```python
from build123d import *

# Parameters (mm, degrees)
CYLINDER100_R               = 6
CYLINDER100_DEPTH           = 9
CYLINDER020_R               = 0.8
CYLINDER020_DEPTH           = 20
ARRAY001006_X_COUNT         = 2
ARRAY001006_X_PITCH         = 22
ARRAY001006_Y_COUNT         = 2
ARRAY001006_Y_PITCH         = 22
ARRAY001006_PLACEMENT_ANGLE = 90
CYLINDER101_R               = 7
CYLINDER101_DEPTH           = 9
BOX008_W                    = 14
BOX008_H                    = 50
BOX008_DEPTH                = 9
FUSION008_ROLL_ANGLE        = 90
FUSION008_PLACEMENT_ANGLE   = 90
CYLINDER106_R               = 2.1
CYLINDER106_DEPTH           = 10
CYLINDER105_R               = 1.85
CYLINDER105_DEPTH           = 20
FUSION009_PLACEMENT_ANGLE   = 90
CYLINDER099_R               = 11.5
CYLINDER099_DEPTH           = 9
BOX_W                       = 9
BOX_H                       = 52
BOX_DEPTH                   = 42
FILLET_R                    = 2


with BuildPart() as lead_hole:
    # Cylinder100 → Cylinder100 (new body)
    with BuildSketch(Plane(origin=(111, 0, 21.5), x_dir=(0, 0, -1), z_dir=(1, 0, 0))):
        Circle(CYLINDER100_R)
    extrude(amount=CYLINDER100_DEPTH)


with BuildPart() as lead_holder_hole_array001:
    # Cylinder020 → Cylinder020 (new body)
    with BuildSketch(Plane.XY):
        Circle(CYLINDER020_R)
    extrude(amount=CYLINDER020_DEPTH)

    # Array001006 X: lead holder hole array001 ×2


with BuildPart() as lead_holder_hole_array001_1:
    add(lead_holder_hole_array001.part)
    with Locations(*[(i * ARRAY001006_X_PITCH, 0, 0) for i in range(1, ARRAY001006_X_COUNT)]):
        add(lead_holder_hole_array001.part)

    # Array001006 Y: lead holder hole array001 ×2


with BuildPart() as lead_holder_hole_array001_2:
    add(lead_holder_hole_array001_1.part)
    with Locations(*[(0, i * ARRAY001006_Y_PITCH, 0) for i in range(1, ARRAY001006_Y_COUNT)]):
        add(lead_holder_hole_array001_1.part)


with BuildPart() as lead_holder_hole_array001_3:
    # Array001006 placement: moved
    add(lead_holder_hole_array001_2.part.moved(Location((111, -11, 32.5))).rotate(Axis((111, -11, 32.5), (0, 1, 0)), ARRAY001006_PLACEMENT_ANGLE))


with BuildPart() as syringe_hole:
    # Cylinder101 → Cylinder101 (new body)
    with BuildSketch(Plane.XY):
        Circle(CYLINDER101_R)
    extrude(amount=CYLINDER101_DEPTH)


with BuildPart() as syringe_hole_fusion:
    # Box008 → Box008 (new body)
    with BuildSketch(Plane(origin=(-7, 0, 0), x_dir=(1, 0, 0), z_dir=(0, 0, 1))):
        with Locations((7, 25)):
            Rectangle(BOX008_W, BOX008_H)
    extrude(amount=BOX008_DEPTH)

    # Fusion008: union syringe_hole
    add(syringe_hole.part)


with BuildPart() as syringe_hole_fusion_1:
    # Fusion008 roll: moved
    add(syringe_hole_fusion.part.rotate(Axis((0, 0, 0), (1, 0, 0)), FUSION008_ROLL_ANGLE))


with BuildPart() as syringe_hole_fusion_2:
    # Fusion008 placement: moved
    add(syringe_hole_fusion_1.part.moved(Location((111, 26, 21.5))).rotate(Axis((111, 26, 21.5), (0, 0, 1)), FUSION008_PLACEMENT_ANGLE))


with BuildPart() as insert_hole001:
    # Cylinder106 → Cylinder106 (new body)
    with BuildSketch(Plane.XY):
        Circle(CYLINDER106_R)
    extrude(amount=CYLINDER106_DEPTH)


with BuildPart() as bolt_insert_hole_fusion:
    # Cylinder105 → Cylinder105 (new body)
    with BuildSketch(Plane.XY.offset(10)):
        Circle(CYLINDER105_R)
    extrude(amount=CYLINDER105_DEPTH)

    # Fusion009: union insert hole001
    add(insert_hole001.part)


with BuildPart() as bolt_insert_hole_fusion_1:
    # Fusion009 placement: moved
    add(bolt_insert_hole_fusion.part.moved(Location((115.5, 12, 31))).rotate(Axis((115.5, 12, 31), (-1, 0, 0)), FUSION009_PLACEMENT_ANGLE))


with BuildPart() as bearing_hole_fusion:
    # Cylinder099 → Cylinder099 (new body)
    with BuildSketch(Plane(origin=(112.4, 0, 21.5), x_dir=(0, 0, -1), z_dir=(1, 0, 0))):
        Circle(CYLINDER099_R)
    extrude(amount=CYLINDER099_DEPTH)

    # Fusion: union lead hole, lead holder hole array001, syringe hole fusion, bolt insert hole fusion
    add(lead_hole.part)
    add(lead_holder_hole_array001_3.part)
    add(syringe_hole_fusion_2.part)
    add(bolt_insert_hole_fusion_1.part)


with BuildPart() as bearing_wall_cut:
    # Box → Box (new body)
    with BuildSketch(Plane(origin=(0, -16, -5), x_dir=(1, 0, 0), z_dir=(0, 0, 1))):
        with Locations((4.5, 26)):
            Rectangle(BOX_W, BOX_H)
    extrude(amount=BOX_DEPTH)

    # Fillet
    fillet_edges = [bearing_wall_cut.edges().sort_by_distance(p)[0] for p in [
        (0, 10, 37),
        (9, 10, 37),
        (4.5, -16, 37),
    ]]
    fillet(fillet_edges, radius=FILLET_R)


with BuildPart() as bearing_wall_cut_1:
    # Compound placement: moved
    add(bearing_wall_cut.part.moved(Location((111, 0, 0))))

    # Cut: cut bearing hole fusion
    add(bearing_hole_fusion.part, mode=Mode.SUBTRACT)


solid = bearing_wall_cut_1.part
```
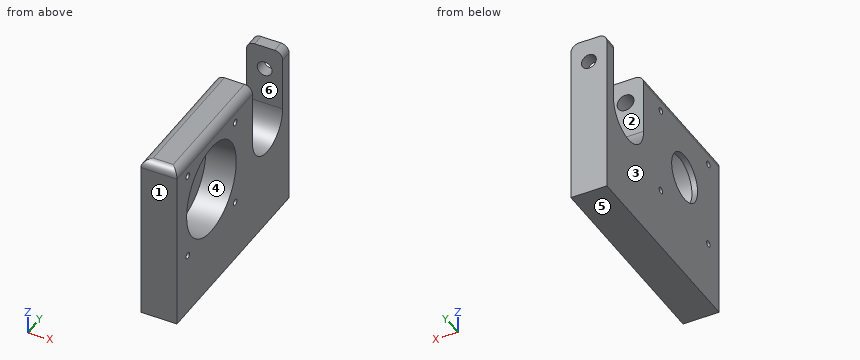
Design review of the part built by this model. Coordinates are the model's own, in mm. Face numbers are marked on the shaded views. A direction names the side the tool comes from. Coordinates: 2 decimals unless noted, no trailing zeros. Loops run counter-clockwise (first coordinate to the right, second up) from the corner with the lowest first, then second, coordinate; pieces in that order, holes last. Notation, with made-up numbers: (-30.5, 20.25) - (11.5, 20.25) arc R32 ccw to (11.5, 46.25) - close; hole circle Ø1 at (-30, 4). An arc over 180 degrees is marked (long way). Use CSV: the item, a comma, the result in double quotes. Start each with the question number.
1) Consider section A-A on x = 115.5. Write out the cut boundary in (y, z).
2) Consider section D-D on z = 31. Write out the cut boundary in (x, y), then the cut area to 3 significant figures.
3) For pin 1 Ø7 at (y, z) = (0, 21.5) entering from -X, flat-tipped, find the tip position at first contact; note if it passes through.
4) Wall thickness on L1, parallel to Z at x = 115.5, y = 34; L2, parallel to Z at x = 115.5, y = 17.5; L3, parallel to Y at x = 112, z = 17.5: over which ranges is each line inside the solid? List them lowest first. Write a range as from..to.
5) Tool access review of the marked faces 4, 5 and 6: name each direction out of +Z, -Z, +X, -X, +Y, -Y from which nothing blocks a thin tool from reaching the whole face with its end or side.
6) Consider section B-B on y = 0. Write out the cut boundary in (x, z).
7) The part is to be moulded in two halves that separate along Y. For the marked faces 1, 2 and 3, say which applies: +Y half, -Y half, draft (parallel to the pull), parting line (faces both ways), or undercut.
8) Consider section C-C on z = 23. Write out the cut boundary in (x, y), then the cut area to 3 significant figures.
Geometry says:
1,outline,"(-16, -5) - (36, -5) - (36, 29.15) - (33, 29.15) - (33, 21.5) arc R7 cw to (19, 21.5) - (19, 28.9) - (12, 28.9) - (12, 33.1) - (19, 33.1) - (19, 37) - (-14, 37) arc R2 ccw to (-16, 35) - close; (33, 32.85) - (36, 32.85) - (36, 37) - (33, 37) - close; hole circle Ø1.6 at (-11, 10.5); hole circle Ø1.6 at (-11, 32.5); hole circle Ø23 at (0, 21.5); hole circle Ø1.6 at (11, 10.5); hole circle Ø1.6 at (11, 32.5)"
2,outline,"(111, -16) - (120, -16) - (120, -6.48) - (112.4, -6.48) - (112.4, 6.48) - (120, 6.48) - (120, 19) - (117.6, 19) - (117.6, 12) - (113.4, 12) - (113.4, 19) - (111, 19) - close; (111, 33) - (113.65, 33) - (113.65, 36) - (111, 36) - close; (117.35, 33) - (120, 33) - (120, 36) - (117.35, 36) - close"
2,area,"203 mm^2"
3,pin 1,"through"
4,L1,"-5..29.15, 32.85..37"
4,L2,"-5..28.9, 33.1..37"
4,L3,"-16..-4.47, 4.47..20.26, 31.74..36"
5,face 4,"+X"
5,face 5,"-Z, +X, -X, +Y, -Y"
5,face 6,"+Z, +X, -X"
6,outline,"(111, -5) - (120, -5) - (120, 10) - (112.4, 10) - (112.4, 15.5) - (111, 15.5) - close; (111, 27.5) - (112.4, 27.5) - (112.4, 33) - (120, 33) - (120, 35) arc R2 ccw to (118, 37) - (113, 37) arc R2 ccw to (111, 35) - close"
7,face 1,"-Y half"
7,face 2,"undercut"
7,face 3,"draft"
8,outline,"(111, -16) - (120, -16) - (120, -11.4) - (112.4, -11.4) - (112.4, -5.81) - (111, -5.81) - close; (111, 5.81) - (112.4, 5.81) - (112.4, 11.4) - (120, 11.4) - (120, 19) - (111, 19) - close; (111, 33) - (120, 33) - (120, 36) - (111, 36) - close"
8,area,"152 mm^2"
